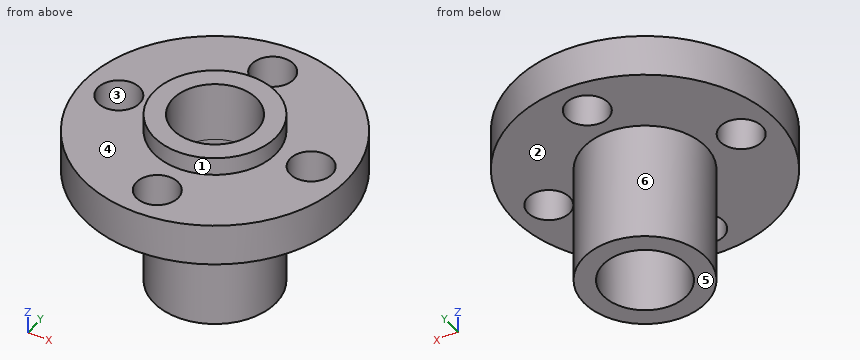
from build123d import *

# Parameters (mm, degrees)
F0_R     = 11
F0_R_2   = 1.75
F0_R_3   = 5.1
F1_DEPTH = 3.5
F0_R_4   = 3.5
F2_DEPTH = 5
F3_DEPTH = 10


with BuildPart() as f1:
    # F0 (on Top) → F1 (new body)
    with BuildSketch(Plane.XY):
        Circle(F0_R)
        with Locations((0, -8)):
            Circle(F0_R_2, mode=Mode.SUBTRACT)
        with Locations((-8, 0)):
            Circle(F0_R_2, mode=Mode.SUBTRACT)
        Circle(F0_R_3, mode=Mode.SUBTRACT)
        with Locations((8, 0)):
            Circle(F0_R_2, mode=Mode.SUBTRACT)
        with Locations((0, 8)):
            Circle(F0_R_2, mode=Mode.SUBTRACT)
    extrude(amount=F1_DEPTH)

    # F0 (on Top) → F2 (join)
    with BuildSketch(Plane.XY):
        Circle(F0_R_3)
        Circle(F0_R_4, mode=Mode.SUBTRACT)
    extrude(amount=F2_DEPTH)

    # F0 (on Top) → F3 (join)
    with BuildSketch(Plane.XY):
        Circle(F0_R_3)
        Circle(F0_R_4, mode=Mode.SUBTRACT)
    extrude(amount=-F3_DEPTH)


solid = f1.part
CAD build for the part. Positions are in the model's coordinates, mm. Face numbers are marked on the shaded views. A direction names the side the tool comes from. Round coordinates to 2 decimals unless told otherwise and drop trailing zeros. Write each loop counter-clockwise with the first axis right and the second up, starting at its lowest first coordinate (ties: lowest second). Pieces come first, ordered by that corner, then holes.
(1) Drop flat-ended pins along their axis: P1, Ø4, axis at x = -8, y = 0, coming from the -Z side; P2, Ø4, axis at x = 0, y = -8, coming from the +Z side; P3, Ø4, axis at x = 0, z = -6, coming from the -Y side. Give the stop position or say it passes through.
(2) Mould opens along Y. For the marked faces 1, 2 and 3 say: pulls with the +Y half, pulls with the -Y half, needs draft (parallel to the pull), parting line crosses it, or undercut.
(3) 3-axis set-ups, long thin cutter, end or side, ignore diameter. For the marked faces 4, 5 and 6: which of +Z, -Z, +X, -X, +Y, -Y reach the whole face in a straight line?
(4) Probe line 1 along Y through (x, z) = (0, 3.4); line 2 along Z through (x, y) = (-3.5, -9.75); line 3 along X through (y, z) = (1.25, -3). List the from-to ranges inside material, lowest first.
(5) Slice it at A-A, the plane y = 0. Write the cut outline in (x, z), and give its area (3 significant figures).
(6) Slice it at C-C, the plane z = -8.5. Write the cut outline in (x, y), and give its area (3 significant figures).
(7) Slice it at D-D, the plane y = -2.25. Write the cut outline in (x, z).
From the geometry:
1. P1: stops at z = 0
1. P2: stops at z = 3.5
1. P3: stops at y = -5.1
2. face 1: parting line crosses it
2. face 2: needs draft
2. face 3: undercut
3. face 4: +Z
3. face 5: -Z, +X, -X, +Y, -Y
3. face 6: -Z
4. line 1: y = -11 to -9.75, -6.25 to -3.5, 3.5 to 6.25, 9.75 to 11
4. line 2: z = 0 to 3.5
4. line 3: x = -4.94 to -3.27, 3.27 to 4.94
5. outline: (-11, 0) - (-9.75, 0) - (-9.75, 3.5) - (-11, 3.5) - close; (-6.25, 0) - (-5.1, 0) - (-5.1, -10) - (-3.5, -10) - (-3.5, 5) - (-5.1, 5) - (-5.1, 3.5) - (-6.25, 3.5) - close; (3.5, -10) - (5.1, -10) - (5.1, 0) - (6.25, 0) - (6.25, 3.5) - (5.1, 3.5) - (5.1, 5) - (3.5, 5) - close; (9.75, 0) - (11, 0) - (11, 3.5) - (9.75, 3.5) - close
5. area: 64.8 mm2
6. outline: circle Ø10.2 at (0, 0); hole circle Ø7 at (0, 0)
6. area: 43.2 mm2
7. outline: (-10.77, 0) - (-4.58, 0) - (-4.58, -10) - (-2.68, -10) - (-2.68, 5) - (-4.58, 5) - (-4.58, 3.5) - (-10.77, 3.5) - close; (2.68, -10) - (4.58, -10) - (4.58, 0) - (10.77, 0) - (10.77, 3.5) - (4.58, 3.5) - (4.58, 5) - (2.68, 5) - close
